```python
from build123d import *

# Parameters (mm, degrees)
F1_DEPTH = 19
F3_D     = 34
F4_W     = 20
F4_H     = 18
F5_DEPTH = 27
F6_W     = 13
F6_H     = 8
F7_DEPTH = 19
F8_W     = 20
F8_H     = 14
F9_DEPTH = 44


with BuildPart() as f1:
    # F0 (on Right) → F1 (new body, symmetric)
    with BuildSketch(Plane.YZ):
        with BuildLine():
            Line((-20.1246117975, 18), (20.1246117975, 18))
            ThreePointArc((20.1246117975, 18), (0, 27), (-20.1246117975, 18))
        make_face()
        with BuildLine():
            ThreePointArc((-20.1246117975, -18), (-27, 0), (-20.1246117975, 18))
            Line((-20.1246117975, 18), (-44, 18))
            Line((-44, 18), (-44, -18))
            Line((-44, -18), (-20.1246117975, -18))
        make_face()
        with BuildLine():
            ThreePointArc((20.1246117975, -18), (25.222653692, -9.6341964239), (27, 0))
            ThreePointArc((27, 0), (25.222653692, 9.6341964239), (20.1246117975, 18))
            Line((20.1246117975, 18), (-20.1246117975, 18))
            ThreePointArc((-20.1246117975, 18), (-27, 0), (-20.1246117975, -18))
            Line((-20.1246117975, -18), (20.1246117975, -18))
        make_face()
        with BuildLine():
            ThreePointArc((20.1246117975, 18), (25.222653692, 9.6341964239), (27, 0))
            ThreePointArc((27, 0), (25.222653692, -9.6341964239), (20.1246117975, -18))
            Line((20.1246117975, -18), (44, -18))
            Line((44, -18), (44, 18))
            Line((44, 18), (20.1246117975, 18))
        make_face()
        with BuildLine():
            ThreePointArc((-20.1246117975, -18), (0, -27), (20.1246117975, -18))
            Line((20.1246117975, -18), (-20.1246117975, -18))
        make_face()
    extrude(amount=F1_DEPTH, both=True)

    # F3 (through all)
    with Locations(Plane.YZ.offset(19)):
        with Locations((0, 0)):
            Hole(F3_D / 2)

    # F4 (on Top) → F5 (cut, symmetric)
    with BuildSketch(Plane.XY):
        Rectangle(F4_W, F4_H)
    extrude(amount=F5_DEPTH, both=True, mode=Mode.SUBTRACT)

    # F6 (on Right) → F7 (cut, symmetric)
    with BuildSketch(Plane.YZ):
        with Locations((-33.5, 0)):
            Rectangle(F6_W, F6_H)
        with Locations((33.5, 0)):
            Rectangle(F6_W, F6_H)
    extrude(amount=F7_DEPTH, both=True, mode=Mode.SUBTRACT)

    # F8 (on Front) → F9 (cut, symmetric)
    with BuildSketch(Plane.XZ):
        Rectangle(F8_W, F8_H)
    extrude(amount=F9_DEPTH, both=True, mode=Mode.SUBTRACT)


solid = f1.part
```
Geometry: final body of the model. Coordinates: model frame, mm. A direction names the side the tool comes from. Coordinates: 2 decimals unless noted, no trailing zeros. Order: outer loops, then holes, each group sorted by start corner. A loop starts at its lowest first (then second) coordinate and runs counter-clockwise, first axis right, second up. Notation, with made-up numbers: M 30.25,67.5 L 78.25,67.5 A20 ccw 78.25,88.5 Z; hole C 4.5,78 d5. An arc over 180 degrees is marked long. Answer in a Markdown table with one row per item. Add a question column.
Q1. Mould query, pull axis Y, two halves, no side actions, for faces 6 (the cylindrical face through (0.27, 9.56, -25.25)), 7 (the flat face through (10, 26, 0)), 8 (the flat face through (-10, 0, 21)). Classes: released by +Y, released by -Y, zero draft, split by the parting line, or undercut.
Q2. Section query B-B on x = 14.5. Return the cut outline in (y, z), and give its area (3 significant figures).
Q3. Line query: L1, parallel to Y at x = 14, z = 0; L2, parallel to Z at x = 5.5, y = 27.5; L3, parallel to Z at x = 14, y = -35.5. Output: solid intervals per line, ascending.
Q4. Section query D-D on x = 2. Return the cut outline in (y, z).
Q5. Section query A-A on z = 0. Count the separate pieces of the cut face and the enclosed holes in it, and give its area (3 significant figures).
Q6. Contact query for flat-ended pins moving along their axis: P1, Ø10, axis at x = -4, y = 34, coming from the -Z side; P2, Ø16, axis at x = -3, y = 31.5, coming from the +Z side; P3, Ø1.5, axis at y = -35, z = 20, coming from the +X side; P4, Ø5, axis at x = -7, y = -20, coming from the +Z side. Output: stop coordinate, or through.
Q7. Reachability of faces 1 (the flat face through (-15, -40, 0)), 2 (the flat face through (0, 30, -7)), 3 (the flat face through (0, 32, -18)), 4 (the flat face through (0, -9, -20)), 5 (the flat face through (19, -1, -18)) from +Z, -Z, +X, -X, +Y, -Y: full face, straight path, thin tool, end or side. Return the list, or none.
Q8. Section query C-C on y = 0. Return the cut outline in (x, z), and give its area (3 significant figures).
Completed:
| question | item | result |
|---|---|---|
| 1 | face 6 | split by the parting line |
| 1 | face 7 | zero draft |
| 1 | face 8 | undercut |
| 2 | outline | M -44,-18 L -20.12,-18 A27 ccw 20.12,-18 L 44,-18 L 44,18 L 20.12,18 A27 ccw -20.12,18 L -44,18 Z; hole M -40,-4 L -27,-4 L -27,4 L -40,4 Z; hole C 0,0 d34; hole M 27,-4 L 40,-4 L 40,4 L 27,4 Z |
| 2 | area | 2,550 mm2 |
| 3 | L1 | y = -44 to -40, -27 to -17, 17 to 27, 40 to 44 |
| 3 | L2 | z = -18 to -7, 7 to 18 |
| 3 | L3 | z = -18 to -4, 4 to 18 |
| 4 | outline | M -44,-18 L -20.12,-18 A27 ccw -9,-25.46 L -9,-14.42 A17 cw -15.49,-7 L -44,-7 Z; M -44,7 L -15.49,7 A17 cw -9,14.42 L -9,25.46 A27 ccw -20.12,18 L -44,18 Z; M 9,-25.46 A27 ccw 20.12,-18 L 44,-18 L 44,-7 L 15.49,-7 A17 cw 9,-14.42 Z; M 9,14.42 A17 cw 15.49,7 L 44,7 L 44,18 L 20.12,18 A27 ccw 9,25.46 Z |
| 5 | separate pieces | 8 |
| 5 | enclosed holes | 0 |
| 5 | area | 504 mm2 |
| 6 | P1 | stops at z = -18 |
| 6 | P2 | stops at z = 18 |
| 6 | P3 | passes through |
| 6 | P4 | stops at z = 20.56 |
| 7 | face 1 | +X, -X |
| 7 | face 2 | +Y, -Y |
| 7 | face 3 | -Z, +X, -X, +Y |
| 7 | face 4 | +Z, -Z |
| 7 | face 5 | +Z, -Z, +X, +Y, -Y |
| 8 | outline | M -19,-27 L -10,-27 L -10,-17 L -19,-17 Z; M -19,17 L -10,17 L -10,27 L -19,27 Z; M 10,-27 L 19,-27 L 19,-17 L 10,-17 Z; M 10,17 L 19,17 L 19,27 L 10,27 Z |
| 8 | area | 360 mm2 |
